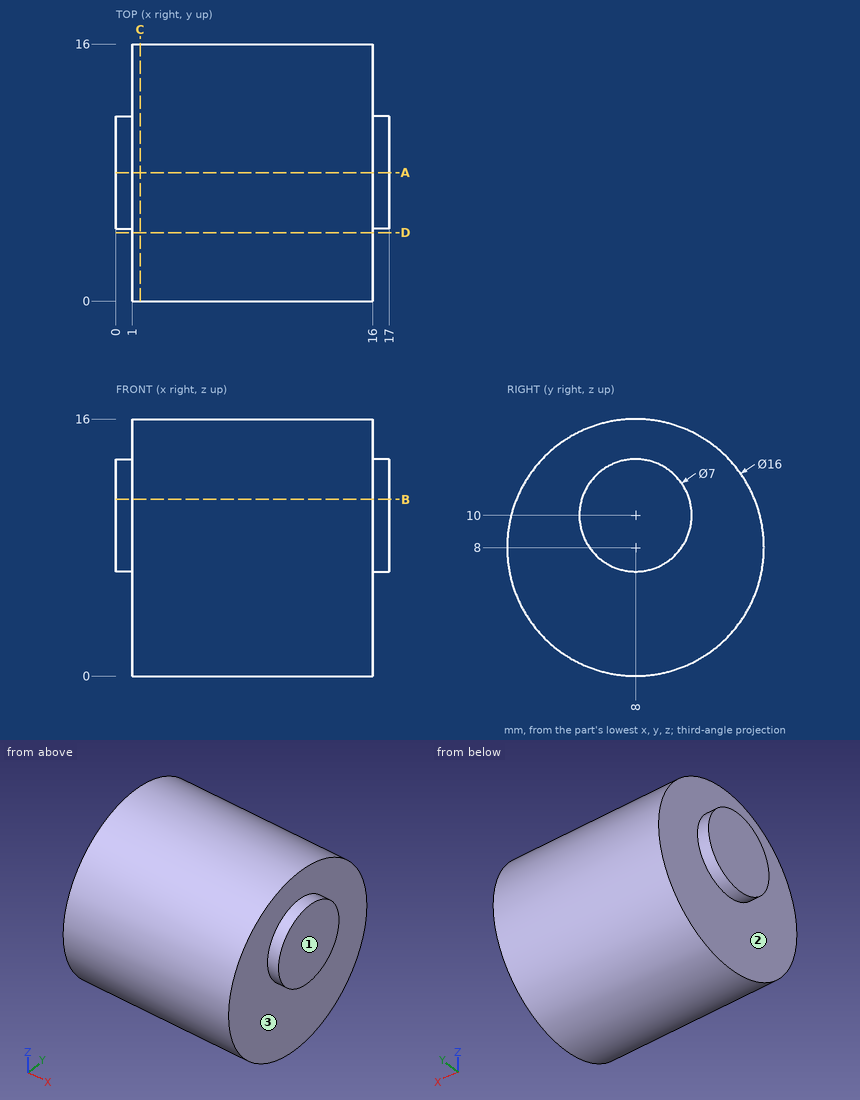
For this review, use the dimensioned drawing (mm, ordinates from the lowest corner) and the shaded views. A direction names the side the tool comes from. Give positions to 0.01 mm unless a question says otherwise; leave off trailing zeros. Loops run counter-clockwise (first coordinate to the right, second up) from the corner with the lowest first, then second, coordinate; pieces in that order, holes last. Notation, with made-up numbers: (-24.5, 43.25) - (-7.5, 43.25) arc R30 ccw to (-7.5, 74.25) - close; hole circle Ø4 at (9, -0.75). An arc over 180 degrees is marked (long way). Write each question's results on one line, items separated by ' | '.
(1) Take a section at B-B (z = 11). Give the boundary of the cut face in (x, y).
Conclusion:
outline: (0, 4.65) - (1, 4.65) - (1, 0.58) - (16, 0.58) - (16, 4.65) - (17, 4.65) - (17, 11.35) - (16, 11.35) - (16, 15.42) - (1, 15.42) - (1, 11.35) - (0, 11.35) - close
(2) For the marked faces 1, 2 and 3, list the 3-axis set-ups (+Z, -Z, +X, -X, +Y, -Y) from which the entire face can be reached by the end or side of a thin tool; tool diameter is ignored.
Conclusion:
face 1: +Z, -Z, +X, +Y, -Y | face 2: -X | face 3: +X
(3) Take a section at A-A (y = 8). Give the boundary of the cut face in (x, z).
Conclusion:
outline: (0, 6.5) - (1, 6.5) - (1, 0) - (16, 0) - (16, 6.5) - (17, 6.5) - (17, 13.5) - (16, 13.5) - (16, 16) - (1, 16) - (1, 13.5) - (0, 13.5) - close
(4) Take a section at D-D (y = 4.25). Give the boundary of the cut face in (x, z), then the cut area to 3 significant figures.
Conclusion:
outline: (1, 0.93) - (16, 0.93) - (16, 15.07) - (1, 15.07) - close | area: 212 mm^2
(5) For pin 1 Ø2 at (x, y) = (7.5, 14) entering from -Z (3 decimals); pin 2 Ø1 at (x, z) = (7, 12) entering from -Y; pin 3 Ø8 at (y, z) = (4, 12) entering from +X; pin 4 Ø4 at (x, z) = (7, 5) entering from -Y, all flat-tipped, find the tip position at first contact; note any pin that passes through.
Conclusion:
pin 1: z = 1.755 | pin 2: y = 0.81 | pin 3: x = 17 | pin 4: y = 0.06
(6) For line 1 along X through (y, z) = (4.5, 6.5); line 2 along Z through (x, y) = (7, 8.25); line 3 along Z through (x, y) = (11.75, 2.25), list the stretches that pass through material, from the lowest coordinate up.
Conclusion:
line 1: 1 to 16 | line 2: 0 to 16 | line 3: 2.44 to 13.56
(7) Take a section at C-C (x = 1.5). Give the boundary of the cut face in (y, z).
Conclusion:
outline: circle Ø16 at (8, 8)
